Design review of the part shown in the three views and the two pictorial views. Dimensions are in mm from the part's minimum x, y and z. A direction names the side the tool comes from. Give positions to 0.01 mm unless a question says otherwise; leave off trailing zeros. Loops run counter-clockwise (first coordinate to the right, second up) from the corner with the lowest first, then second, coordinate; pieces in that order, holes last.
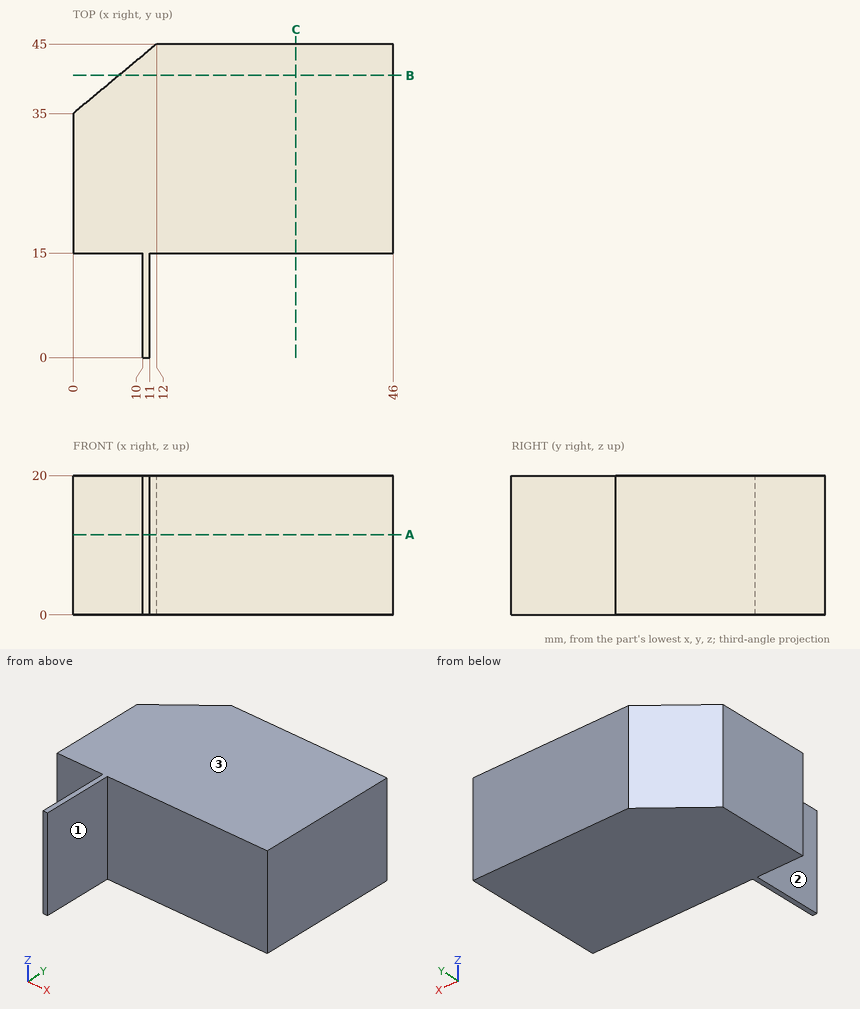
Q1. For pin 1 Ø3 at (x, z) = (7.5, 12.5) entering from -Y; pin 2 Ø7.5 at (y, z) = (5.5, 7.5) entering from -X; pin 3 Ø7.5 at (y, z) = (6.5, 13.5) entering from +X, all flat-tipped, find the tip position at first contact; note any pin that passes through.
Answers:
pin 1: stops at y = 15
pin 2: stops at x = 10
pin 3: stops at x = 11
Q2. Consider section B-B on y = 40.5. Give the boundary of the cut face in (x, z).
Answers:
outline: (6.6, 0) - (46, 0) - (46, 20) - (6.6, 20) - close
Q3. Consider section A-A on z = 11.5. Give the boundary of the cut face in (x, y).
Answers:
outline: (0, 15) - (10, 15) - (10, 0) - (11, 0) - (11, 15) - (46, 15) - (46, 45) - (12, 45) - (0, 35) - close
Q4. For probe 1 along X at (y, z) = (2, 3.75); probe 2 along Y at (x, z) = (32.5, 4.75); probe 3 along Y at (x, z) = (4.5, 17.75), list the stretches that pass through material, from the lowest coordinate up.
Answers:
probe 1: x = 10 to 11
probe 2: y = 15 to 45
probe 3: y = 15 to 38.75
Q5. Machinability: for the marked faces 1, 2 and 3, which of the approach directions +Z, -Z, +X, -X, +Y, -Y give a long, thin tool a straight path to every point of the face, cutting with its end or side? Answer none if there is none.
Answers:
face 1: +Z, -Z, +X, -Y
face 2: +Z, -Z, -X, -Y
face 3: +Z, +X, -X, +Y, -Y
Q6. Consider section C-C on x = 32. Give the boundary of the cut face in (y, z), plus the area to 3 significant figures.
Answers:
outline: (15, 0) - (45, 0) - (45, 20) - (15, 20) - close
area: 600 mm2
